from build123d import *

# Parameters (mm, degrees)
CROQUIS2_W              = 70
CROQUIS2_H              = 40
SALIENTE_EXTRUIR1_DEPTH = 45
CROQUIS3_W              = 40.5
CROQUIS3_H              = 20
CORTAR_EXTRUIR1_DEPTH   = 39
CROQUIS4_W              = 7
CROQUIS4_H              = 20
CORTAR_EXTRUIR2_DEPTH   = 12
CROQUIS5_W              = 20
CROQUIS5_H              = 20
CORTAR_EXTRUIR4_DEPTH   = 7
CROQUIS6_R              = 7.5
SALIENTE_EXTRUIR3_DEPTH = 30
CROQUIS8_R              = 7.5
SALIENTE_EXTRUIR4_DEPTH = 30
CROQUIS9_W              = 30
CROQUIS9_H              = 40
SALIENTE_EXTRUIR5_DEPTH = 10
CROQUIS10_R             = 10
SALIENTE_EXTRUIR6_DEPTH = 54
REDONDEO1_R             = 5


with BuildPart() as part:
    # Croquis2 → Saliente-Extruir1 (new body)
    with BuildSketch(Plane.XY):
        with Locations((35, 20)):
            Rectangle(CROQUIS2_W, CROQUIS2_H)
    extrude(amount=SALIENTE_EXTRUIR1_DEPTH)

    # Croquis3 → Cortar-Extruir1 (cut)
    with BuildSketch(Plane(origin=(0, 0, 0), x_dir=(-1, 0, 0), z_dir=(0, 0, -1))):
        with Locations((-27.25, 20)):
            Rectangle(CROQUIS3_W, CROQUIS3_H)
    extrude(amount=-CORTAR_EXTRUIR1_DEPTH, mode=Mode.SUBTRACT)

    # Croquis4 → Cortar-Extruir2 (cut)
    with BuildSketch(Plane(origin=(0, 0, 0), x_dir=(-1, 0, 0), z_dir=(0, 0, -1))):
        with Locations((-3.5, 20)):
            Rectangle(CROQUIS4_W, CROQUIS4_H)
        with Locations((-51, 20)):
            Rectangle(CROQUIS4_W, CROQUIS4_H)
    extrude(amount=-CORTAR_EXTRUIR2_DEPTH, mode=Mode.SUBTRACT)

    # Croquis5 → Cortar-Extruir4 (cut)
    with BuildSketch(Plane.ZY):
        with Locations((35, 20)):
            Rectangle(CROQUIS5_W, CROQUIS5_H)
    extrude(amount=-CORTAR_EXTRUIR4_DEPTH, mode=Mode.SUBTRACT)

    # Croquis6 → Saliente-Extruir3 (add)
    with BuildSketch(Plane(origin=(0, 40, 0), x_dir=(1, 0, 0), z_dir=(0, 1, 0))):
        with Locations((52.5, -22.5)):
            Circle(CROQUIS6_R)
    extrude(amount=SALIENTE_EXTRUIR3_DEPTH)

    # Croquis8 → Saliente-Extruir4 (add)
    with BuildSketch(Plane.XZ):
        with Locations((52.5, 22.5)):
            Circle(CROQUIS8_R)
    extrude(amount=SALIENTE_EXTRUIR4_DEPTH)

    # Croquis9 → Saliente-Extruir5 (add)
    with BuildSketch(Plane(origin=(0, 0, 0), x_dir=(-1, 0, 0), z_dir=(0, 0, -1))):
        with Locations((-15, 20)):
            Rectangle(CROQUIS9_W, CROQUIS9_H)
    extrude(amount=SALIENTE_EXTRUIR5_DEPTH)

    # Croquis10 → Saliente-Extruir6 (add)
    with BuildSketch(Plane(origin=(0, 0, -10), x_dir=(-1, 0, 0), z_dir=(0, 0, -1))):
        with Locations((-15, 20)):
            Circle(CROQUIS10_R)
    extrude(amount=SALIENTE_EXTRUIR6_DEPTH)

    # Redondeo1
    redondeo1_edges = [part.edges().sort_by_distance(p)[0] for p in [
        (70, 20, 0),
    ]]
    fillet(redondeo1_edges, radius=REDONDEO1_R)


solid = part.part
Could you check a few things on this model? Use its own coordinates, in mm. A direction names the side the tool comes from. Give positions to 0.01 mm unless a question says otherwise; leave off trailing zeros. Order: outer loops, then holes, each group sorted by start corner. A loop starts at its lowest first (then second) coordinate and runs counter-clockwise, first axis right, second up. Notation, with made-up numbers: (-16, 21.25) -> (-11, 21.25) arc R16 cw to (-11, 49.25) -> close; hole circle Ø5 at (-5, -4.5). An arc over 180 degrees is marked (long way). Answer in a Markdown table with one row per item. Add a question column.
Item 1: Imagine slicing it at A-A (y = 20). List the corners of the cut face in (x, z) for me, and give its area (3 significant figures).
Item 2: Imagine slicing it at D-D (y = 36.5). List the corners of the cut face in (x, z) for me, and give its area (3 significant figures).
Item 3: We'd pull the mould along Y, two halves only. Please class faces 5 (the flat face through (52, 70, 22)), 6 (the flat face through (7, 20, 42)), 7 (the flat face through (35, 20, 45)), 8 (the flat face through (28, 30, 17)): pulls with the +Y half, pulls with the -Y half, needs draft (parallel to the pull), parting line crosses it, or undercut.
Item 4: For faces 1 (the cylindrical face through (51.524, -14.79, 29.936)), 2 (the flat face through (47.5, 20, 25)), 3 (the flat face through (55, 20, 0)), 4 (the cylindrical face through (51.524, 54.79, 15.064)), which set-ups out of +Z, -Z, +X, -X, +Y, -Y let a thin tool reach every point of the face, with its end or its side?
Item 5: Please list where these lines run through material, in increasing order: probe 1 along Z at (x, y) = (59, 8); probe 2 along Y at (x, z) = (15.5, -41); probe 3 along Y at (x, z) = (9, 10.5).
Item 6: Imagine slicing it at B-B (z = 22.5). List the corners of the cut face in (x, y) for me.
Item 7: I'm going to push flat-ended pins straight in: P1, Ø3, axis at y = 21, z = 40.5, coming from the -X side; P2, Ø22.5, axis at x = 23, z = 14.5, coming from the +Y side; P3, Ø2, axis at x = 7.5, z = -39.5, coming from the -Y side. Where does each tip first touch, or does it pass through?
Item 8: Imagine slicing it at C-C (x = 28.5). List the corners of the cut face in (y, z) for me, and give its area (3 significant figures).
Result:
| question | item | result |
|---|---|---|
| 1 | outline | (0, -10) -> (5, -10) -> (5, -64) -> (25, -64) -> (25, -10) -> (30, -10) -> (30, 0) -> (0, 0) -> close; (0, 12) -> (7, 12) -> (7, 25) -> (0, 25) -> close; (7, 39) -> (47.5, 39) -> (47.5, 12) -> (54.5, 12) -> (54.5, 0) -> (65, 0) arc R5 ccw to (70, 5) -> (70, 45) -> (7, 45) -> close |
| 1 | area | 2,640 mm2 |
| 2 | outline | (0, -10) -> (30, -10) -> (30, 0) -> (65, 0) arc R5 ccw to (70, 5) -> (70, 45) -> (0, 45) -> close |
| 2 | area | 3,440 mm2 |
| 3 | face 5 | pulls with the +Y half |
| 3 | face 6 | undercut |
| 3 | face 7 | needs draft |
| 3 | face 8 | undercut |
| 4 | face 1 | -Y |
| 4 | face 2 | -Z |
| 4 | face 3 | -Z, +X, +Y, -Y |
| 4 | face 4 | +Y |
| 5 | probe 1 | 0 to 45 |
| 5 | probe 2 | 10.01 to 29.99 |
| 5 | probe 3 | 0 to 10, 30 to 40 |
| 6 | outline | (0, 0) -> (45, 0) -> (45, -30) -> (60, -30) -> (60, 0) -> (70, 0) -> (70, 40) -> (60, 40) -> (60, 70) -> (45, 70) -> (45, 40) -> (0, 40) -> close; hole (7, 10) -> (47.5, 10) -> (47.5, 30) -> (7, 30) -> close |
| 7 | P1 | x = 7 |
| 7 | P2 | y = 40 |
| 7 | P3 | y = 12.4 |
| 8 | outline | (0, -10) -> (40, -10) -> (40, 45) -> (0, 45) -> close; hole (10, 0) -> (30, 0) -> (30, 39) -> (10, 39) -> close |
| 8 | area | 1,420 mm2 |
